from build123d import *

# Parameters (mm, degrees)
CROQUIS1_R              = 35
SALIENTE_EXTRUIR1_DEPTH = 47.6
CROQUIS2_W              = 81.100238634
CROQUIS2_H              = 55.229590233
CORTAR_EXTRUIR1_DEPTH   = 69.671391423
CROQUIS3_W              = 90
CROQUIS3_H              = 10
SALIENTE_EXTRUIR2_DEPTH = 47.6
CROQUIS4_R              = 2.5
CORTAR_EXTRUIR2_DEPTH   = 75.268162762
CROQUIS5_R              = 20
CORTAR_EXTRUIR3_DEPTH   = 75.268162762
REDONDEO1_R             = 10
CORTAR_EXTRUIR4_START   = -6.8
CROQUIS6_R              = 27.5
CORTAR_EXTRUIR4_DEPTH   = 37
CORTAR_EXTRUIR5_START   = 10
CROQUIS7_R              = 30
CORTAR_EXTRUIR5_DEPTH   = 17


with BuildPart() as part:
    # Croquis1 → Saliente-Extruir1 (new body)
    with BuildSketch(Plane.XY):
        Circle(CROQUIS1_R)
    extrude(amount=SALIENTE_EXTRUIR1_DEPTH)

    # Croquis2 → Cortar-Extruir1 (cut, through all)
    with BuildSketch(Plane.XY.offset(47.6)):
        with Locations((5.550119317, 27.614795117)):
            Rectangle(CROQUIS2_W, CROQUIS2_H)
    extrude(amount=-CORTAR_EXTRUIR1_DEPTH, mode=Mode.SUBTRACT)

    # Croquis3 → Saliente-Extruir2 (add)
    with BuildSketch(Plane.XY.offset(47.6)):
        with Locations((0, -5)):
            Rectangle(CROQUIS3_W, CROQUIS3_H)
    extrude(amount=-SALIENTE_EXTRUIR2_DEPTH)

    # Croquis4 → Cortar-Extruir2 (cut, through all)
    with BuildSketch(Plane(origin=(0, 0, 0), x_dir=(1, 0, 0), z_dir=(0, 1, 0))):
        with Locations(Location((39, -9.8, 0), (0, 0, 270))):
            Circle(CROQUIS4_R)
        with Locations(Location((39, -37.8, 0), (0, 0, 90))):
            Circle(CROQUIS4_R)
        with Locations(Location((-39, -37.8, 0), (0, 0, 270))):
            Circle(CROQUIS4_R)
        with Locations(Location((-39, -9.8, 0), (0, 0, 90))):
            Circle(CROQUIS4_R)
    extrude(amount=-CORTAR_EXTRUIR2_DEPTH, mode=Mode.SUBTRACT)

    # Croquis5 → Cortar-Extruir3 (cut, through all)
    with BuildSketch(Plane(origin=(0, 0, 0), x_dir=(-1, 0, 0), z_dir=(0, 0, -1))):
        Circle(CROQUIS5_R)
    extrude(amount=-CORTAR_EXTRUIR3_DEPTH, mode=Mode.SUBTRACT)

    # Redondeo1
    redondeo1_edges = [part.edges().sort_by_distance(p)[0] for p in [
        (-45, -5, 47.6),
        (45, -5, 47.6),
        (-45, -5, 0),
        (45, -5, 0),
    ]]
    fillet(redondeo1_edges, radius=REDONDEO1_R)

    # Croquis6 → Cortar-Extruir4 (cut)
    with BuildSketch(Plane.XY.offset(47.6).offset(CORTAR_EXTRUIR4_START)):
        Circle(CROQUIS6_R)
    extrude(amount=-CORTAR_EXTRUIR4_DEPTH, mode=Mode.SUBTRACT)

    # Croquis7 → Cortar-Extruir5 (cut)
    with BuildSketch(Plane(origin=(0, 0, 40.8), x_dir=(-1, 0, 0), z_dir=(0, 0, -1)).offset(CORTAR_EXTRUIR5_START)):
        Circle(CROQUIS7_R)
    extrude(amount=CORTAR_EXTRUIR5_DEPTH, mode=Mode.SUBTRACT)


solid = part.part
Geometry: final body of the model. Coordinates: model frame, mm. A direction names the side the tool comes from. Give positions to 0.01 mm unless a question says otherwise; leave off trailing zeros. Order: outer loops, then holes, each group sorted by start corner. A loop starts at its lowest first (then second) coordinate and runs counter-clockwise, first axis right, second up. Notation, with made-up numbers: (-8, 37.5) -> (48, 37.5) arc R14 cw to (48, 52.5) -> close; hole circle Ø10 at (1.5, -17.75). An arc over 180 degrees is marked (long way). Answer as a JSON object with one key per item and string values.
Q1. Section A-A (y = -2). State how many separate pieces and enclosed holes the cut face has, plus the area to 3 significant figures.
Entries:
{"separate pieces": "2", "enclosed holes": "4", "area": "1,580 mm^2"}
Q2. Draft query along X for faces 1 (the flat face through (45, -5, 24)), 2 (the cylindrical face through (0, -20, 44)), 3 (the flat face through (0, -21, 47.6)). Return one class per face: released by +X, released by -X, zero draft, split by the parting line, or undercut.
Entries:
{"face 1": "released by +X", "face 2": "undercut", "face 3": "zero draft"}
Q3. Section C-C (z = 39). Output: boundary loops of the cut face in (x, y).
Entries:
{"outline": "(-44.9, -10) -> (-41.19, -10) -> (-41.19, 0) -> (-44.9, 0) -> close; (-36.81, -10) -> (-33.54, -10) arc R35 ccw to (33.54, -10) -> (36.81, -10) -> (36.81, 0) -> (27.5, 0) arc R27.5 cw to (-27.5, 0) -> (-36.81, 0) -> close; (41.19, -10) -> (44.9, -10) -> (44.9, 0) -> (41.19, 0) -> close"}
Q4. Section D-D (y = -25.5). Output: boundary loops of the cut face in (x, z), plus the area to 3 significant figures.
Entries:
{"outline": "(-23.97, 0) -> (23.97, 0) -> (23.97, 47.6) -> (-23.97, 47.6) -> close; hole (-15.8, 13.8) -> (-10.3, 13.8) -> (-10.3, 3.8) -> (10.3, 3.8) -> (10.3, 13.8) -> (15.8, 13.8) -> (15.8, 30.8) -> (10.3, 30.8) -> (10.3, 40.8) -> (-10.3, 40.8) -> (-10.3, 30.8) -> (-15.8, 30.8) -> close", "area": "1,330 mm^2"}
Q5. First-contact query: pin 1 (4 mm diameter, centred on x = -5, z = 33.5, fed in from +Y); pin 2 (12.5 mm diameter, centred on x = -38, z = 24.5, fed in from -Y); pin 3 (12.5 mm diameter, centred on x = 40, z = 20.5, fed in from -Y). Flat tips, straight axial feed; report the tip coordinate or a pass-through.
Entries:
{"pin 1": "stops at y = -26.59", "pin 2": "stops at y = -14.73", "pin 3": "stops at y = -10"}
Q6. Section B-B (x = 0). Output: boundary loops of the cut face in (y, z), plus the area to 3 significant figures.
Entries:
{"outline": "(-35, 0) -> (-20, 0) -> (-20, 3.8) -> (-27.5, 3.8) -> (-27.5, 13.8) -> (-30, 13.8) -> (-30, 30.8) -> (-27.5, 30.8) -> (-27.5, 40.8) -> (-20, 40.8) -> (-20, 47.6) -> (-35, 47.6) -> close", "area": "394 mm^2"}
Q7. Access query for faces 4 (the flat face through (-39, -10, 24)), 5 (the cylindrical face through (-0.605, -27.493, 8.87)), 6 (the cylindrical face through (38.9, -4.9, 40.3)), 7 (the flat face through (39, -10, 24)). Directions: +Z, -Z, +X, -X, +Y, -Y. A direction counts if a zero-diameter tool reaches every point of the face in a straight line with its end or side. Return the directions, or none.
Entries:
{"face 4": "+Z, -Z, -X, -Y", "face 5": "+Y", "face 6": "+Y, -Y", "face 7": "+Z, -Z, +X, -Y"}
Q8. Material intervals for probe 1 along Z at (x, y) = (-10, -17.5); probe 2 along X at (y, z) = (-5, 37); probe 3 along X at (y, z) = (-3, 37), sorted ascending.
Entries:
{"probe 1": "z = 0 to 3.8, 40.8 to 47.6", "probe 2": "x = -45 to -41.37, -36.63 to -27.04, 27.04 to 36.63, 41.37 to 45", "probe 3": "x = -45 to -41.37, -36.63 to -27.34, 27.34 to 36.63, 41.37 to 45"}
